```python
from build123d import *

# Parameters (mm, degrees)
EXTRUDE_1_DEPTH        = 3
SKETCH_3_R             = 16
SKETCH_3_R_2           = 2.25
SKETCH_3_R_3           = 5
CUT_EXTRUDE_3_DEPTH    = 417.901436616
EXTRUDE_START          = -3
EXTRUDE_4_DEPTH        = 3
SKETCH_5_R             = 1.75
CUT_EXTRUDE_5_DEPTH    = 433.011573919
PATTERN_LINEAR_1_COUNT = 4
PATTERN_LINEAR_1_PITCH = 70


with BuildPart() as part:
    # 草圖1 → 伸長1 (new body)
    with BuildSketch(Plane.XY):
        with BuildLine():
            Line((55.280581326, 100), (374.719418674, 100))
            ThreePointArc((374.719418674, 100), (401.086913014, 84.309271198), (399.872727163, 53.650349482))
            Line((399.872727163, 53.650349482), (373.872727163, 13.650349482))
            ThreePointArc((373.872727163, 13.650349482), (363.028689873, 3.63250566), (348.719418674, 0))
            Line((348.719418674, 0), (81.280581326, 0))
            ThreePointArc((81.280581326, 0), (66.971310127, 3.63250566), (56.127272837, 13.650349482))
            Line((56.127272837, 13.650349482), (30.127272837, 53.650349482))
            ThreePointArc((30.127272837, 53.650349482), (28.913086986, 84.309271198), (55.280581326, 100))
        make_face()
    extrude(amount=EXTRUDE_1_DEPTH)

    # 草圖3 → 伸長3 (cut, through all)
    with BuildSketch(Plane.XY.offset(3)):
        with Locations((55.280581326, 70)):
            Circle(SKETCH_3_R)
        with Locations((55.280581326, 90)):
            Circle(SKETCH_3_R_2)
        with Locations((75.280581326, 70)):
            Circle(SKETCH_3_R_2)
        with Locations((55.280581326, 50)):
            Circle(SKETCH_3_R_2)
        with Locations((35.280581326, 70)):
            Circle(SKETCH_3_R_2)
        with Locations((374.719418674, 70)):
            Circle(SKETCH_3_R_3)
    extrude(amount=-CUT_EXTRUDE_3_DEPTH, mode=Mode.SUBTRACT)

    # 草圖4 → 伸長4 (add)
    with BuildSketch(Plane.XY.offset(3).offset(EXTRUDE_START)):
        with BuildLine():
            Line((399.872727163, 53.650349482), (391, 40))
            Line((391, 40), (415, 40))
            Line((415, 40), (415, 120))
            Line((415, 120), (15, 120))
            Line((15, 120), (15, 40))
            Line((15, 40), (39, 40))
            Line((39, 40), (30.127272837, 53.650349482))
            ThreePointArc((30.127272837, 53.650349482), (28.913086986, 84.309271198), (55.280581326, 100))
            Line((55.280581326, 100), (374.719418674, 100))
            ThreePointArc((374.719418674, 100), (401.086913014, 84.309271198), (399.872727163, 53.650349482))
        make_face()
    extrude(amount=EXTRUDE_4_DEPTH)

    # 草圖5 → 伸長5 (cut, through all)
    with BuildSketch(Plane.XY.offset(3)):
        with Locations((130, 30)):
            Circle(SKETCH_5_R)
        with Locations((90, 30)):
            Circle(SKETCH_5_R)
    cut_extrude_5 = extrude(amount=-CUT_EXTRUDE_5_DEPTH, mode=Mode.SUBTRACT)

    # 直線複製排列1: 伸長5 ×4
    with Locations(*[(i * PATTERN_LINEAR_1_PITCH, 0, 0) for i in range(1, PATTERN_LINEAR_1_COUNT)]):
        add(cut_extrude_5, mode=Mode.SUBTRACT)


solid = part.part
```
CAD build for the part. Positions are in the model's coordinates, mm. Coordinates: 2 decimals unless noted, no trailing zeros. Loops run counter-clockwise (first coordinate to the right, second up) from the corner with the lowest first, then second, coordinate; pieces in that order, holes last. Notation, with made-up numbers: (-27.5, 11) - (2.5, 11) arc R22 cw to (2.5, 20) - close; hole circle Ø9 at (81.25, 5). An arc over 180 degrees is marked (long way). Return JSON: item names as keys, results as strings.
1. Drop a flat-ended pin along its axis: pin 1 (3 mm diameter, centred on x = 340, y = 30, fed in from +Z). Give the stop position or say it passes through.
Result:
{"pin 1": "passes through"}
2. Band-saw the part on B-B (x = 385.5). Give the cut face in (y, z), and give its area (3 significant figures).
Result:
{"outline": "(31.54, 0) - (120, 0) - (120, 3) - (31.54, 3) - close", "area": "265 mm2"}
3. Mould opens along X. For faces 1 (the flat face through (212, 61, 3)), 2 (the cylindrical face through (67.16, 3.53, 1.48)), 3 (the cylindrical face through (53.198, 85.864, 1.521)) say: released by +X, released by -X, zero draft, split by the parting line, or undercut.
Result:
{"face 1": "zero draft", "face 2": "released by -X", "face 3": "undercut"}
4. Probe L1, parallel to X at y = 67, z = 1.8; L2, parallel to Y at x = 200, z = 1.4; L3, parallel to X at y = 88, z = 2.45. List the from-to ranges inside material, lowest first. Write a range as from..to.
Result:
{"L1": "x = 15..39.56, 71..370.72, 378.72..415", "L2": "y = 0..28.25, 31.75..120", "L3": "x = 15..54.25, 56.31..415"}
5. Band-saw the part on A-A (z = 1.9). State how many separate pieces and enclosed holes the cut face has, and give its area (3 significant figures).
Result:
{"separate pieces": "1", "enclosed holes": "14", "area": "43,900 mm2"}
